Autodesk Inventor part; units mm, degrees
ref_plane "C1_XY" through (0, 0, 0) normal (0, 0, 1) x (1, 0, 0)
ref_plane "C1_YZ" through (0, 0, 0) normal (1, 0, 0) x (0, 1, 0)
ref_plane "C1_ZX" through (0, 0, 0) normal (0, 1, 0) x (0, 0, 1)
sketch "Sketch_1" plane through (0, 0, 0) normal (0, 0, 1) x (1, 0, 0)
  line L0 (-15, -4) -> (-15, -13)
  arc A0 (-15, -13) -> (-13, -15) centre (-13, -13) ccw
  line L1 (-13, -15) -> (-4, -15)
  line L2 (-4, -15) -> (-4, -13)
  line L3 (-4, -13) -> (-8.25, -13)
  line L4 (-8.25, -13) -> (-8.25, -9.6642)
  line L5 (-8.25, -9.6642) -> (-4.5858, -6)
  line L6 (-4.5858, -6) -> (-0.5196, -6)
  line L7 (-0.5196, -6) -> (0, -5.7)
  line L8 (0, -5.7) -> (0.5196, -6)
  line L9 (0.5196, -6) -> (4.5858, -6)
  line L10 (4.5858, -6) -> (8.25, -9.6642)
  line L11 (8.25, -9.6642) -> (8.25, -13)
  line L12 (8.25, -13) -> (4, -13)
  line L13 (4, -13) -> (4, -15)
  line L14 (4, -15) -> (13, -15)
  arc A1 (13, -15) -> (15, -13) centre (13, -13) ccw
  line L15 (15, -13) -> (15, -4)
  line L16 (15, -4) -> (13, -4)
  line L17 (13, -4) -> (13, -8.25)
  line L18 (13, -8.25) -> (9.6642, -8.25)
  line L19 (9.6642, -8.25) -> (6, -4.5858)
  line L20 (6, -4.5858) -> (6, -0.5196)
  line L21 (6, -0.5196) -> (5.7, 0)
  line L22 (5.7, 0) -> (6, 0.5196)
  line L23 (6, 0.5196) -> (6, 4.5858)
  line L24 (6, 4.5858) -> (9.6642, 8.25)
  line L25 (9.6642, 8.25) -> (13, 8.25)
  line L26 (13, 8.25) -> (13, 4)
  line L27 (13, 4) -> (15, 4)
  line L28 (15, 4) -> (15, 13)
  arc A2 (15, 13) -> (13, 15) centre (13, 13) ccw
  line L29 (13, 15) -> (4, 15)
  line L30 (4, 15) -> (4, 13)
  line L31 (4, 13) -> (8.25, 13)
  line L32 (8.25, 13) -> (8.25, 9.6642)
  line L33 (8.25, 9.6642) -> (4.5858, 6)
  line L34 (4.5858, 6) -> (0.5196, 6)
  line L35 (0.5196, 6) -> (0, 5.7)
  line L36 (0, 5.7) -> (-0.5196, 6)
  line L37 (-0.5196, 6) -> (-4.5858, 6)
  line L38 (-4.5858, 6) -> (-8.25, 9.6642)
  line L39 (-8.25, 9.6642) -> (-8.25, 13)
  line L40 (-8.25, 13) -> (-4, 13)
  line L41 (-4, 13) -> (-4, 15)
  line L42 (-4, 15) -> (-13, 15)
  arc A3 (-13, 15) -> (-15, 13) centre (-13, 13) ccw
  line L43 (-15, 13) -> (-15, 4)
  line L44 (-15, 4) -> (-13, 4)
  line L45 (-13, 4) -> (-13, 8.25)
  line L46 (-13, 8.25) -> (-9.6642, 8.25)
  line L47 (-9.6642, 8.25) -> (-6, 4.5858)
  line L48 (-6, 4.5858) -> (-6, 0.5196)
  line L49 (-6, 0.5196) -> (-5.7, 0)
  line L50 (-5.7, 0) -> (-6, -0.5196)
  line L51 (-6, -0.5196) -> (-6, -4.5858)
  line L52 (-6, -4.5858) -> (-9.6642, -8.25)
  line L53 (-9.6642, -8.25) -> (-13, -8.25)
  line L54 (-13, -8.25) -> (-13, -4)
  line L55 (-13, -4) -> (-15, -4)
extrude "Extrusion1" add sketch "Sketch_1" against normal blind 140
sketch "Sketch2" plane through (0, 0, -140) normal (0, 0, -1) x (-1, 0, 0)
  point P0 (0, 0)
hole "Hole1" at (0, 0, -140) direction (0, 0, 1) diameter 6.8 depth 140
sketch "Sketch3" plane through (0, 0, -140) normal (0, 0, -1) x (-1, 0, 0)
  point P0 (-11.6, 11.6)
hole "Hole2" at (11.6, 11.6, -140) direction (0, 0, 1) diameter 4.2 depth 140
pattern_linear "Rectangular Pattern1" count 2 spacing 23.2 along (-1, 0, 0) count 2 spacing 23.2 along (0, -1, 0) of "Hole2"
ref_plane "C1_XY" through (0, 0, 0) normal (0, 0, 1) x (1, 0, 0)
ref_plane "C1_YZ" through (0, 0, 0) normal (1, 0, 0) x (0, 1, 0)
ref_plane "C1_ZX" through (0, 0, 0) normal (0, 1, 0) x (0, 0, 1)
ref_plane "to_frame_cap1_XY" through (0, 0, 0) normal (0, 0, 1) x (1, 0, 0)
ref_plane "to_frame_cap1_YZ" through (0, 0, 0) normal (1, 0, 0) x (0, 1, 0)
ref_plane "to_frame_cap1_ZX" through (0, 0, 0) normal (0, 1, 0) x (0, 0, 1)
ref_plane "to_frame_cap2_XY" through (0, 0, -140) normal (0, 0, -1) x (1, 0, 0)
ref_plane "to_frame_cap2_YZ" through (0, 0, -140) normal (1, 0, 0) x (0, -1, 0)
ref_plane "to_frame_cap2_ZX" through (0, 0, -140) normal (0, -1, 0) x (0, 0, -1)
properties part number "HFS6-3030-140"
Source: CAD feature listing. Evaluate the final solid. Frame: model axes, mm. A direction names the side the tool comes from. Give positions to 0.01 mm unless a question says otherwise; leave off trailing zeros. Loops run counter-clockwise (first coordinate to the right, second up) from the corner with the lowest first, then second, coordinate; pieces in that order, holes last. Notation, with made-up numbers: (77, 57) -> (115, 57) arc R24 ccw to (115, 90) -> close; hole circle Ø1 at (-8, 6). An arc over 180 degrees is marked (long way). Use a Markdown table: item, result. Add a question column.
(1) Section query A-A (x = -11.6). Output: boundary loops of the cut face in (y, z), then the cut area to 3 significant figures.
(2) Section query C-C (z = -27.5). Count the separate pieces of the cut face and the enclosed holes in it, then the cut area to 3 significant figures.
(3) Access query for faces 4 (the face through (11, 8.25, -69)), 5 (the face through (15, -9, -69)). Directions: +Z, -Z, +X, -X, +Y, -Y. A direction counts if a zero-diameter tool reaches every point of the face in a straight line with its end or side. Return the directions, or none.
(4) Pull-direction query (X, two-part tool) for faces 1 (the face through (-3, -6, -69)), 2 (the face through (-4, 0, 0)), 3 (the face through (15, 8, -69)); classes: +X half, -X half, draft (parallel to the pull), parting line (faces both ways), or undercut.
(5) Ray query, line 1 (X direction, y = 11.6, z = -69.5); line 2 (X direction, y = 5.25, z = -126). Return the intervals inside material, ascending.
(6) First-contact query: pin 1 Ø0.6 at (y, z) = (-14, -53) entering from +X; pin 2 Ø1 at (y, z) = (14, -39.5) entering from -X; pin 3 Ø1.2 at (y, z) = (2, -99) entering from +X. Flat tips, straight axial feed; report the tip coordinate or a pass-through.
Checked values:
| question | item | result |
|---|---|---|
| 1 | outline | (-15, -140) -> (-13.7, -140) -> (-13.7, 0) -> (-15, 0) -> close; (-9.5, -140) -> (-8.25, -140) -> (-8.25, 0) -> (-9.5, 0) -> close; (8.25, -140) -> (9.5, -140) -> (9.5, 0) -> (8.25, 0) -> close; (13.7, -140) -> (15, -140) -> (15, 0) -> (13.7, 0) -> close |
| 1 | area | 714 mm^2 |
| 2 | separate pieces | 1 |
| 2 | enclosed holes | 5 |
| 2 | area | 332 mm^2 |
| 3 | face 4 | +Z, -Z |
| 3 | face 5 | +Z, -Z, +X, +Y, -Y |
| 4 | face 1 | undercut |
| 4 | face 2 | draft |
| 4 | face 3 | +X half |
| 5 | line 1 | -15 to -13.7, -9.5 to -8.25, 8.25 to 9.5, 13.7 to 15 |
| 5 | line 2 | -15 to -13, -6.66 to 6.66, 13 to 15 |
| 6 | pin 1 | x = 14.87 |
| 6 | pin 2 | x = -14.94 |
| 6 | pin 3 | x = 6 |
